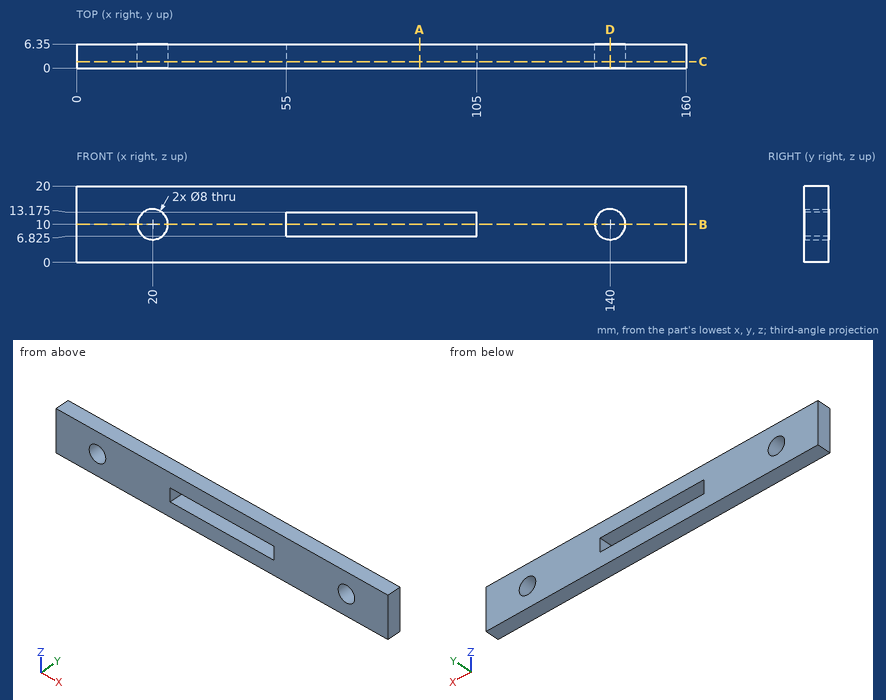
The figure shows three views and two pictorial views of one solid part (mm, origin at its lowest corner). Answer the questions. Give positions to 0.01 mm unless a question says otherwise; leave off trailing zeros. Write each loop counter-clockwise with the first axis right and the second up, starting at its lowest first coordinate (ties: lowest second). Pieces come first, ordered by that corner, then holes. Notation, with made-up numbers: (19, 65.25) - (29, 65.25) arc R22 ccw to (29, 84.25) - close; hole circle Ø5 at (83.5, 74.25). An arc over 180 degrees is marked (long way). Use one line per item in the form item = value. Start each with the question number.
1) Find section C-C on y = 1.75. Determine the outline of the cut face in (x, z) (3 decimals).
2) Find section A-A on x = 90. Determine the outline of the cut face in (y, z) (3 decimals), plus the area to 3 significant figures.
3) Find section D-D on x = 140. Determine the outline of the cut face in (y, z).
4) A flat-ended cylindrical pin translates along its axis: pin 1 Ø1 at (x, z) = (94, 11.5) entering from -Y. Find the tip coordinate at first contact, or state that the pin passes through.
5) Find section B-B on z = 10. Determine the outline of the cut face in (x, y).
6) Consider line 1 along Z through (x, y) = (79.5, 6.25) (3 decimals); line 2 along Z through (x, y) = (20, 2.25). Determine where each line is inside the solid, lowest interval first. Write a range as from..to.
Geometry results:
q1.outline = (0, 0) - (160, 0) - (160, 20) - (0, 20) - close; hole circle Ø8 at (20, 10); hole (55, 6.825) - (105, 6.825) - (105, 13.175) - (55, 13.175) - close; hole circle Ø8 at (140, 10)
q2.outline = (0, 0) - (6.35, 0) - (6.35, 6.825) - (0, 6.825) - close; (0, 13.175) - (6.35, 13.175) - (6.35, 20) - (0, 20) - close
q2.area = 86.7 mm2
q3.outline = (0, 0) - (6.35, 0) - (6.35, 6) - (0, 6) - close; (0, 14) - (6.35, 14) - (6.35, 20) - (0, 20) - close
q4.pin_1 = through
q5.outline = (0, 0) - (16, 0) - (16, 6.35) - (0, 6.35) - close; (24, 0) - (55, 0) - (55, 6.35) - (24, 6.35) - close; (105, 0) - (136, 0) - (136, 6.35) - (105, 6.35) - close; (144, 0) - (160, 0) - (160, 6.35) - (144, 6.35) - close
q6.line_1 = 0..6.825, 13.175..20
q6.line_2 = 0..6, 14..20
